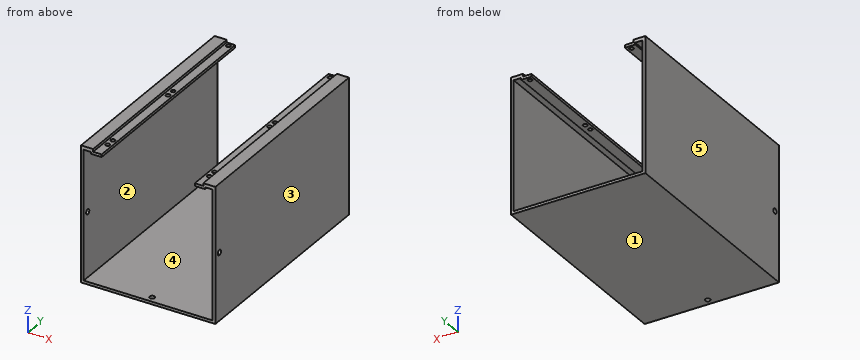
```python
from build123d import *

# Parameters (mm, degrees)
BOSS_EXTRUDE1_DEPTH = 327.5
SKETCH2_R           = 1.6
CUT_EXTRUDE2_DEPTH  = 10
SKETCH3_R           = 1.93
CUT_EXTRUDE3_DEPTH  = 102
SKETCH4_R           = 1.93
CUT_EXTRUDE4_DEPTH  = 10
SKETCH5_W           = 116.752499477
SKETCH5_H           = 165.661363519
CUT_EXTRUDE5_DEPTH  = 191
SKETCH6_W           = 83
SKETCH6_H           = 2.003
CUT_EXTRUDE6_DEPTH  = 203


with BuildPart() as part:
    # Sketch1 → Boss-Extrude1 (new body)
    with BuildSketch(Plane(origin=(0, 0, 0), x_dir=(1, 0, 0), z_dir=(0, 1, 0))):
        Polygon((0, -0.603), (0, 101.206), (101.206, 101.206), (101.206, -0.6), (91.5, -0.6), (91.5, 1.4), (85.703, 1.4), (85.703, 3.4), (93.5, 3.4), (93.5, 2), (99.206, 2), (99.206, 99.206), (2, 99.206), (2, 2), (7.706, 2), (7.706, 3.397), (15.503, 3.397), (15.503, 1.397), (9.706, 1.397), (9.706, -0.603), align=None)
    extrude(amount=BOSS_EXTRUDE1_DEPTH)

    # Sketch2 → Cut-Extrude2 (cut)
    with BuildSketch(Plane.XY.offset(-1.397)):
        with Locations((12.303, 314.9)):
            Circle(SKETCH2_R)
        with Locations((12.303, 308.5)):
            Circle(SKETCH2_R)
        with Locations((88.903, 314.9)):
            Circle(SKETCH2_R)
        with Locations((88.903, 308.5)):
            Circle(SKETCH2_R)
        with Locations((12.303, 240.925)):
            Circle(SKETCH2_R)
        with Locations((12.303, 234.525)):
            Circle(SKETCH2_R)
        with Locations((88.903, 240.925)):
            Circle(SKETCH2_R)
        with Locations((88.903, 234.525)):
            Circle(SKETCH2_R)
        with Locations((12.303, 166.95)):
            Circle(SKETCH2_R)
        with Locations((12.303, 160.55)):
            Circle(SKETCH2_R)
        with Locations((88.903, 166.95)):
            Circle(SKETCH2_R)
        with Locations((88.903, 160.55)):
            Circle(SKETCH2_R)
        with Locations((12.303, 92.975)):
            Circle(SKETCH2_R)
        with Locations((12.303, 86.575)):
            Circle(SKETCH2_R)
        with Locations((88.903, 92.975)):
            Circle(SKETCH2_R)
        with Locations((88.903, 86.575)):
            Circle(SKETCH2_R)
        with Locations((12.303, 19)):
            Circle(SKETCH2_R)
        with Locations((12.303, 12.6)):
            Circle(SKETCH2_R)
        with Locations((88.903, 19)):
            Circle(SKETCH2_R)
        with Locations((88.903, 12.6)):
            Circle(SKETCH2_R)
    extrude(amount=-CUT_EXTRUDE2_DEPTH, mode=Mode.SUBTRACT)

    # Sketch3 → Cut-Extrude3 (cut)
    with BuildSketch(Plane(origin=(101.206, 0, 0), x_dir=(0, 0, -1), z_dir=(1, 0, 0))):
        with Locations((50.603, 322.524)):
            Circle(SKETCH3_R)
        with Locations((50.603, 4.976)):
            Circle(SKETCH3_R)
    extrude(amount=-CUT_EXTRUDE3_DEPTH, mode=Mode.SUBTRACT)

    # Sketch4 → Cut-Extrude4 (cut)
    with BuildSketch(Plane(origin=(0, 0, -101.206), x_dir=(-1, 0, 0), z_dir=(0, 0, -1))):
        with Locations((-50.603, 322.524)):
            Circle(SKETCH4_R)
        with Locations((-50.603, 4.976)):
            Circle(SKETCH4_R)
    extrude(amount=-CUT_EXTRUDE4_DEPTH, mode=Mode.SUBTRACT)

    # Sketch5 → Cut-Extrude5 (cut)
    with BuildSketch(Plane.ZY):
        with Locations((-42.829750262, 246.58068176)):
            Rectangle(SKETCH5_W, SKETCH5_H)
    extrude(amount=-CUT_EXTRUDE5_DEPTH, mode=Mode.SUBTRACT)

    # Sketch6 → Cut-Extrude6 (cut)
    with BuildSketch(Plane(origin=(0, 163.75, 0), x_dir=(1, 0, 0), z_dir=(0, 1, 0))):
        with Locations((50.603, 0.3985)):
            Rectangle(SKETCH6_W, SKETCH6_H)
    extrude(amount=-CUT_EXTRUDE6_DEPTH, mode=Mode.SUBTRACT)


solid = part.part
```
Design review of the part built by this model. Coordinates are the model's own, in mm. Face numbers are marked on the shaded views. A direction names the side the tool comes from. Round coordinates to 2 decimals unless told otherwise and drop trailing zeros. Order: outer loops, then holes, each group sorted by start corner. A loop starts at its lowest first (then second) coordinate and runs counter-clockwise, first axis right, second up. Notation, with made-up numbers: (-37, 15.5) - (11, 15.5) arc R14 cw to (11, 24.5) - close; hole circle Ø11 at (-4, 81.5). An arc over 180 degrees is marked (long way). Return JSON: item names as keys, results as strings.
Q1. Machinability: for the marked faces 1 and 2, which of the approach directions +Z, -Z, +X, -X, +Y, -Y give a long, thin tool a straight path to every point of the face, cutting with its end or side? Answer none if there is none.
Computed values:
{"face 1": "-Z, +X, -X, +Y, -Y", "face 2": "+Y, -Y"}
Q2. Consider section C-C on x = 36. Write out the cut boundary in (y, z).
Computed values:
{"outline": "(0, -101.21) - (163.75, -101.21) - (163.75, -99.21) - (0, -99.21) - close"}
Q3. Consider section B-B on y = 126. Write out the cut boundary in (x, z), plus the area to 3 significant figures.
Computed values:
{"outline": "(0, -101.21) - (101.21, -101.21) - (101.21, 0.6) - (92.1, 0.6) - (92.1, -1.4) - (85.7, -1.4) - (85.7, -3.4) - (93.5, -3.4) - (93.5, -2) - (99.21, -2) - (99.21, -99.21) - (2, -99.21) - (2, -2) - (7.71, -2) - (7.71, -3.4) - (15.5, -3.4) - (15.5, -1.4) - (9.1, -1.4) - (9.1, 0.6) - (0, 0.6) - close", "area": "668 mm2"}
Q4. Consider section A-A on z = -86.5. Write out the cut boundary in (x, y), plus the area to 3 significant figures.
Computed values:
{"outline": "(0, 0) - (2, 0) - (2, 163.75) - (0, 163.75) - close; (99.21, 0) - (101.21, 0) - (101.21, 163.75) - (99.21, 163.75) - close", "area": "655 mm2"}
Q5. Wall thickness on L1, parallel to X at y = 56, z = -22.5; L2, parallel to Z at x = 6.5, y = 55; L3, parallel to Z at x = 87.5, y = 85.5: over which ranges is each line inside the solid? List them lowest first. Write a range as [from, to].
Computed values:
{"L1": "x = [0, 2], [99.21, 101.21]", "L2": "z = [-101.21, -99.21], [-2, 0.6]", "L3": "z = [-101.21, -99.21], [-3.4, -1.4]"}
Q6. The part is to be moulded in two halves that separate along X. For the marked faces 3, 4 and 5, say which applies: pulls with the +X half, pulls with the -X half, needs draft (parallel to the pull), parting line crosses it, or undercut.
Computed values:
{"face 3": "pulls with the +X half", "face 4": "undercut", "face 5": "pulls with the -X half"}
Q7. For pin 1 Ø5 at (x, y) = (56, 132) entering from +Z; pin 2 Ø1.9 at (x, y) = (11, 92.5) entering from +Z; pin 3 Ø3.5 at (y, z) = (4.976, -50.603) entering from +X, all flat-tipped, find the tip position at first contact; note any pin that passes through.
Computed values:
{"pin 1": "stops at z = -99.21", "pin 2": "stops at z = -1.4", "pin 3": "passes through"}
